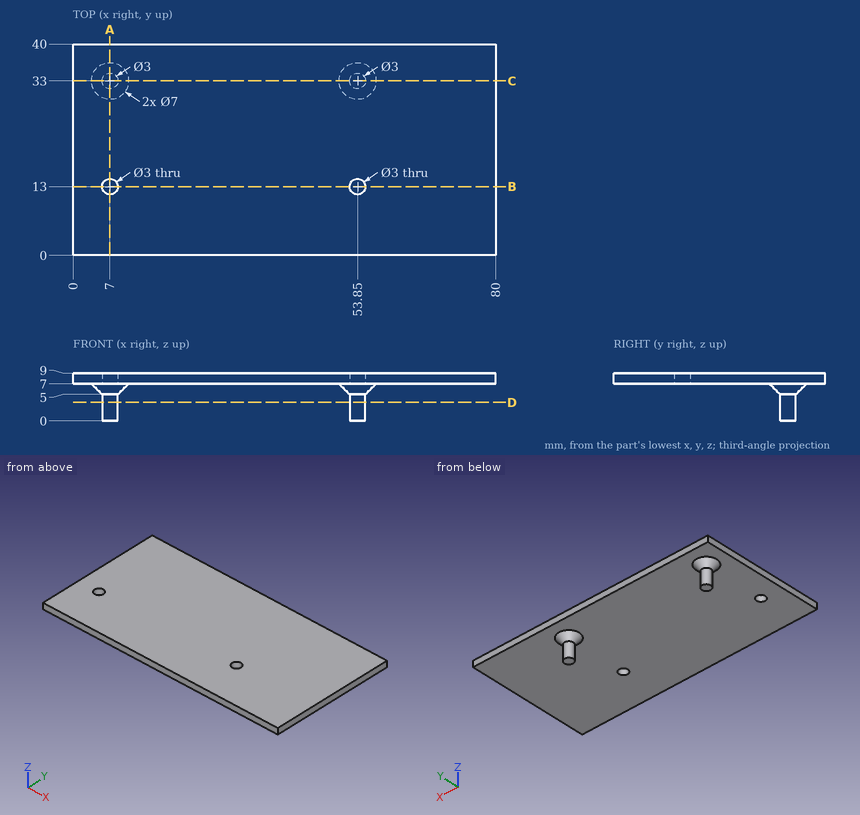
Drawing for the job (mm, zero at the part's lowest x, y, z). Round coordinates to 2 decimals unless told otherwise and drop trailing zeros. Loops run counter-clockwise (first coordinate to the right, second up) from the corner with the lowest first, then second, coordinate; pieces in that order, holes last. Notation, with made-up numbers: (13.25, 67.25) - (62.25, 67.25) arc R31 cw to (62.25, 97.25) - close; hole circle Ø8 at (20.5, -34.5). An arc over 180 degrees is marked (long way). Return JSON: item names as keys, results as strings. Group by question number.
Q1. Drill centre lines: line 1 along X through (y, z) = (13, 7.6); line 2 along Y through (x, z) = (7, 7.4); line 3 along Z through (x, y) = (17, 13.5). Where is each one in solid material? Low to high. Write a range as [from, to].
Q2. Band-saw the part on A-A on x = 7. Give the cut face in (y, z), plus the area to 3 significant figures.
Q3. Band-saw the part on D-D on z = 3.5. Give the cut face in (x, y), plus the area to 3 significant figures.
Q4. Flat gauge pins, fed straight in: pin 1 Ø1.5 at (y, z) = (14, 6.5) entering from +X; pin 2 Ø1 at (x, y) = (11.5, 9) entering from -Z. Where does each tip first touch, or does it go through?
Q5. Band-saw the part on C-C on y = 33. Give the cut face in (x, z).
Q6. Band-saw the part on B-B on y = 13. Give the cut face in (x, z), plus the area to 3 significant figures.
Solutions:
{
 "1": {"line 1": "x = [0, 5.5], [8.5, 52.35], [55.35, 80]", "line 2": "y = [0, 11.5], [14.5, 40]", "line 3": "z = [7, 9]"},
 "2": {"outline": "(0, 7) - (11.5, 7) - (11.5, 9) - (0, 9) - close; (14.5, 7) - (29.5, 7) - (31.5, 5) - (31.5, 0) - (34.5, 0) - (34.5, 5) - (36.5, 7) - (40, 7) - (40, 9) - (14.5, 9) - close", "area": "99.0 mm^2"},
 "3": {"outline": "circle Ø3 at (7, 33); circle Ø3 at (53.85, 33)", "area": "14.1 mm^2"},
 "4": {"pin 1": "stops at x = 80", "pin 2": "stops at z = 7"},
 "5": {"outline": "(0, 7) - (3.5, 7) - (5.5, 5) - (5.5, 0) - (8.5, 0) - (8.5, 5) - (10.5, 7) - (50.35, 7) - (52.35, 5) - (52.35, 0) - (55.35, 0) - (55.35, 5) - (57.35, 7) - (80, 7) - (80, 9) - (0, 9) - close"},
 "6": {"outline": "(0, 7) - (5.5, 7) - (5.5, 9) - (0, 9) - close; (8.5, 7) - (52.35, 7) - (52.35, 9) - (8.5, 9) - close; (55.35, 7) - (80, 7) - (80, 9) - (55.35, 9) - close", "area": "148 mm^2"}
}
